Could you check a few things on this model? Use its own coordinates, in mm. Coordinates: 2 decimals unless noted, no trailing zeros. Order: outer loops, then holes, each group sorted by start corner. A loop starts at its lowest first (then second) coordinate and runs counter-clockwise, first axis right, second up. Notation, with made-up numbers: (46.25, 27.25) -> (51.25, 27.25) arc R18 cw to (51.25, 52.25) -> close; hole circle Ø1 at (-24, 27). An arc over 180 degrees is marked (long way). Put each result on its own line as item: value. Start each with the question number.
Q1. If we section it at D-D (x = 12.5): Please give me the cut outline in (y, z).
Q2. Will this pin go through, and if not, where does the flat tip stop? pin 1 (1.2 mm diameter, centred on x = -6.5, y = 1, fed in from +Z).
Q3. If we section it at C-C (x = 0): Please give me the cut outline in (y, z).
Q4. If we section it at B-B (y = 3.1): Please give me the cut outline in (x, z).
Q5. If we section it at A-A (z = 0): Please give me the cut outline in (x, y), and give its area (3 significant figures).
Q6. Please list where these lines run through material, in increasing order: line 1 along Z through (x, y) = (0, 2.4); line 2 along X through (y, z) = (2.05, 21); line 3 along Z through (x, y) = (15, 0.7).
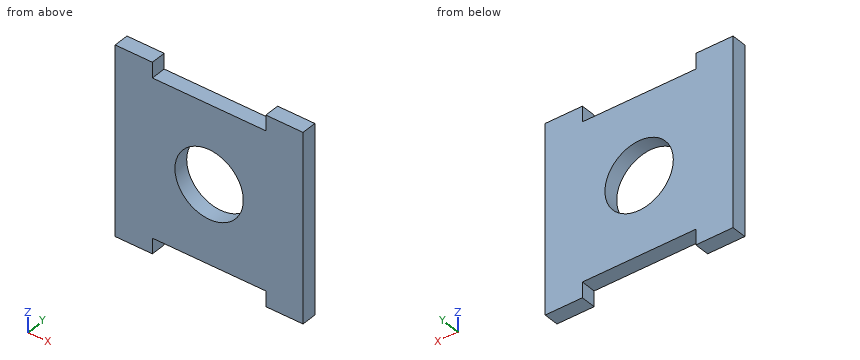
Autodesk Inventor part; units mm, degrees
ref_plane "YZ Plane" through (0, 0, 0) normal (1, 0, 0) x (0, 1, 0)
ref_plane "XZ Plane" through (0, 0, 0) normal (0, 1, 0) x (-1, 0, 0)
ref_plane "XY Plane" through (0, 0, 0) normal (0, 0, 1) x (1, 0, 0)
sketch "스케치1" plane through (0, 0, 0) normal (0, 1, 0) x (-1, 0, 0)
  line L0 (25, 25) -> (-25, 25)
  line L1 (-25, 25) -> (-25, -25)
  line L2 (-25, -25) -> (25, -25)
  line L3 (25, -25) -> (25, 25)
  circle A0 centre (0, 0) radius 9.1
  line L4 (15.1, 25) -> (15.1, 20.9)
  line L5 (15.1, 20.9) -> (-15.1, 20.9)
  line L6 (-15.1, 20.9) -> (-15.1, 25)
  line L7 (15.1, -25) -> (15.1, -20.9)
  line L8 (15.1, -20.9) -> (-15.1, -20.9)
  line L9 (-15.1, -20.9) -> (-15.1, -25)
  point P0 (15.1, 22.95)
  point P1 (15.1, -22.95)
  dimension "d0" = 25
  dimension "d2" = 25
  dimension "d3" = 25
  dimension "d4" = 25
  dimension "d5" = 18.2
  dimension "d6" = 30.2
  dimension "d7" = 30.2
  dimension "d8" = 9.9
  dimension "d9" = 9.9
  dimension "d10" = 4.1
  dimension "d11" = 4.1
extrude "돌출1" add sketch "스케치1" along normal blind 4 contours L3 L2 L7 L8 L9 L1 L0 L6 L5 L4
properties part number "센서 마운트"
The answers:
1. outline: (0, -20.9) -> (4, -20.9) -> (4, 20.9) -> (0, 20.9) -> close
2. pin 1: z = 20.9
3. outline: (0, -20.9) -> (4, -20.9) -> (4, -9.1) -> (0, -9.1) -> close; (0, 9.1) -> (4, 9.1) -> (4, 20.9) -> (0, 20.9) -> close
4. outline: (-25, -25) -> (-15.1, -25) -> (-15.1, -20.9) -> (15.1, -20.9) -> (15.1, -25) -> (25, -25) -> (25, 25) -> (15.1, 25) -> (15.1, 20.9) -> (-15.1, 20.9) -> (-15.1, 25) -> (-25, 25) -> close; hole circle Ø18.2 at (0, 0)
5. outline: (-25, 0) -> (-9.1, 0) -> (-9.1, 4) -> (-25, 4) -> close; (9.1, 0) -> (25, 0) -> (25, 4) -> (9.1, 4) -> close
5. area: 127 mm^2
6. line 1: -20.9 to -9.1, 9.1 to 20.9
6. line 2: -25 to -15.1, 15.1 to 25
6. line 3: -20.9 to 20.9
